```python
from build123d import *

# Parameters (mm, degrees)
SKETCH_R    = 16
PAD_DEPTH   = 20
FILLET_R    = 3
FILLET001_R = 3
FILLET002_R = 3
FILLET003_R = 3
FILLET004_R = 3
FILLET005_R = 3
FILLET006_R = 3
FILLET007_R = 3


with BuildPart() as part:
    # Sketch → Pad (new body)
    with BuildSketch(Plane.XY):
        with BuildLine():
            ThreePointArc((3, -21.794495), (15.556349, -15.556349), (21.794495, -3))
            Line((21.794495, -3), (38.132171, -3))
            ThreePointArc((38.132171, -3), (38.25, 0), (38.132171, 3))
            Line((38.132171, 3), (21.794495, 3))
            ThreePointArc((21.794495, 3), (15.556349, 15.556349), (3, 21.794495))
            Line((3, 21.794495), (3, 38.132171))
            ThreePointArc((3, 38.132171), (0, 38.25), (-3, 38.132171))
            Line((-3, 38.132171), (-3, 21.794495))
            ThreePointArc((-3, 21.794495), (-15.556349, 15.556349), (-21.794495, 3))
            Line((-21.794495, 3), (-38.132171, 3))
            ThreePointArc((-38.132171, 3), (-38.25, 0), (-38.132171, -3))
            Line((-38.132171, -3), (-21.794495, -3))
            ThreePointArc((-21.794495, -3), (-15.556349, -15.556349), (-3, -21.794495))
            Line((-3, -21.794495), (-3, -38.132171))
            ThreePointArc((-3, -38.132171), (0, -38.25), (3, -38.132171))
            Line((3, -38.132171), (3, -21.794495))
        make_face()
        Circle(SKETCH_R, mode=Mode.SUBTRACT)
    extrude(amount=PAD_DEPTH)

    # Fillet
    fillet_edges = [part.edges().sort_by_distance(p)[0] for p in [
        (3, -21.794495, 10),
    ]]
    fillet(fillet_edges, radius=FILLET_R)

    # Fillet001
    fillet001_edges = [part.edges().sort_by_distance(p)[0] for p in [
        (21.794495, -3, 10),
    ]]
    fillet(fillet001_edges, radius=FILLET001_R)

    # Fillet002
    fillet002_edges = [part.edges().sort_by_distance(p)[0] for p in [
        (-3, -21.794495, 10),
    ]]
    fillet(fillet002_edges, radius=FILLET002_R)

    # Fillet003
    fillet003_edges = [part.edges().sort_by_distance(p)[0] for p in [
        (-21.794495, -3, 10),
    ]]
    fillet(fillet003_edges, radius=FILLET003_R)

    # Fillet004
    fillet004_edges = [part.edges().sort_by_distance(p)[0] for p in [
        (-21.794495, 3, 10),
    ]]
    fillet(fillet004_edges, radius=FILLET004_R)

    # Fillet005
    fillet005_edges = [part.edges().sort_by_distance(p)[0] for p in [
        (-3, 21.794495, 10),
    ]]
    fillet(fillet005_edges, radius=FILLET005_R)

    # Fillet006
    fillet006_edges = [part.edges().sort_by_distance(p)[0] for p in [
        (3, 21.794495, 10),
    ]]
    fillet(fillet006_edges, radius=FILLET006_R)

    # Fillet007
    fillet007_edges = [part.edges().sort_by_distance(p)[0] for p in [
        (21.794495, 3, 10),
    ]]
    fillet(fillet007_edges, radius=FILLET007_R)


solid = part.part
```
CAD build for the part. Positions are in the model's coordinates, mm. A direction names the side the tool comes from. Give positions to 0.01 mm unless a question says otherwise; leave off trailing zeros. Order: outer loops, then holes, each group sorted by start corner. A loop starts at its lowest first (then second) coordinate and runs counter-clockwise, first axis right, second up.
(1) Flat gauge pins, fed straight in: pin 1 (10 mm diameter, centred on x = 28, z = 16.5, fed in from +Y); pin 2 (11 mm diameter, centred on y = 34, z = 12, fed in from +X); pin 3 (12 mm diameter, centred on x = -10.5, z = 15, fed in from -Y). Where does each tip first touch, or does it go through?
(2) Saw through at D-D, the plane y = 33.5. Give the cut face in (x, z), then the cut area to 3 significant figures.
(3) Tool access for faces 1 (the flat face through (-3, -31, 10)), 2 (the flat face through (31, 3, 10)), 3 (the flat face through (3, -31, 10)): list every direction of +Z, -Z, +X, -X, +Y, -Y with a clear straight run to the whole face (end or side of a thin tool).
(4) Saw through at C-C, the plane z = 15. Give the cut face in (x, y).
(5) Drill centre lines: L1, parallel to Y at x = 0, z = 12; L2, parallel to X at y = 29.5, z = 1; L3, parallel to X at y = 13.5, z = 8.5. Where is each one in solid material? Low to high.
(6) Mould opens along X. For faces 4 (the cylindrical face through (-3.47, -15.62, 9.86)), 5 (the cylindrical face through (15.67, 15.44, 9.86)), 6 (the cylindrical face through (-22.44, 3.62, 10.14)), 7 (the flat face through (31, -3, 10)) say: released by +X, released by -X, zero draft, split by the parting line, or undercut.
(7) Saw through at A-A, the plane x = 0. Give the cut face in (y, z), then the cut area to 3 significant figures.
Results found:
1. pin 1: stops at y = 3.28
1. pin 2: stops at x = 3
1. pin 3: stops at y = -21.67
2. outline: (-3, 0) - (3, 0) - (3, 20) - (-3, 20) - close
2. area: 120 mm2
3. face 1: +Z, -Z, -X, -Y
3. face 2: +Z, -Z, +X, +Y
3. face 3: +Z, -Z, +X, -Y
4. outline: (-38.13, -3) - (-24.27, -3) arc R3 cw to (-21.36, -5.28) arc R22 ccw to (-5.28, -21.36) arc R3 cw to (-3, -24.27) - (-3, -38.13) arc R38.25 ccw to (3, -38.13) - (3, -24.27) arc R3 cw to (5.28, -21.36) arc R22 ccw to (21.36, -5.28) arc R3 cw to (24.27, -3) - (38.13, -3) arc R38.25 ccw to (38.13, 3) - (24.27, 3) arc R3 cw to (21.36, 5.28) arc R22 ccw to (5.28, 21.36) arc R3 cw to (3, 24.27) - (3, 38.13) arc R38.25 ccw to (-3, 38.13) - (-3, 24.27) arc R3 cw to (-5.28, 21.36) arc R22 ccw to (-21.36, 5.28) arc R3 cw to (-24.27, 3) - (-38.13, 3) arc R38.25 ccw to start; hole circle Ø32 at (0, 0)
5. L1: y = -38.25 to -16, 16 to 38.25
5. L2: x = -3 to 3
5. L3: x = -17.37 to -8.59, 8.59 to 17.37
6. face 4: undercut
6. face 5: released by +X
6. face 6: released by -X
6. face 7: zero draft
7. outline: (-38.25, 0) - (-16, 0) - (-16, 20) - (-38.25, 20) - close; (16, 0) - (38.25, 0) - (38.25, 20) - (16, 20) - close
7. area: 890 mm2
